Design review of the part shown in the three views and the two pictorial views. Dimensions are in mm from the part's minimum x, y and z. Coordinates: 2 decimals unless noted, no trailing zeros. Loops run counter-clockwise (first coordinate to the right, second up) from the corner with the lowest first, then second, coordinate; pieces in that order, holes last. Notation, with made-up numbers: M -26.75,68.5 L -1.75,68.5 A25 cw -1.75,87.5 Z; hole C 86,-33 d6. An arc over 180 degrees is marked long. Answer as a JSON object with one key per item and string values. Group by question number.
Item 1: Wall thickness on L1, parallel to X at y = 58.5, z = 42.5: over which ranges is the line inside the solid? List them lowest first. Write a range as from..to.
Item 2: Add section A-A (x = 12.5). State the section outline as (y, z) points, then the cut area to 3 significant figures.
Item 3: Add section C-C (z = 40). State the section outline as (x, y) points, then the cut area to 3 significant figures.
Item 4: Add section B-B (y = 29). State the section outline as (x, z) points, then the cut area to 3 significant figures.
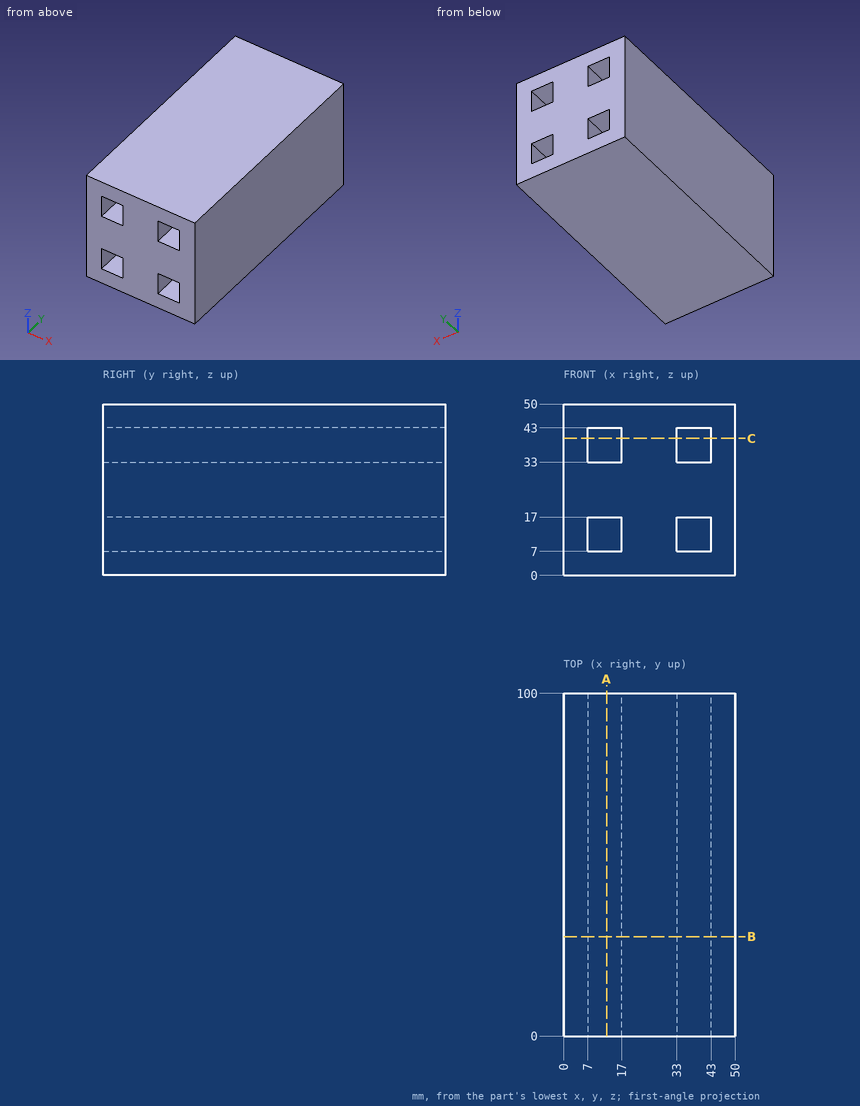
From the geometry:
{
 "1": {"L1": "x = 0..7, 17..33, 43..50"},
 "2": {"outline": "M 0,0 L 100,0 L 100,7 L 0,7 Z; M 0,17 L 100,17 L 100,33 L 0,33 Z; M 0,43 L 100,43 L 100,50 L 0,50 Z", "area": "3,000 mm²"},
 "3": {"outline": "M 0,0 L 7,0 L 7,100 L 0,100 Z; M 17,0 L 33,0 L 33,100 L 17,100 Z; M 43,0 L 50,0 L 50,100 L 43,100 Z", "area": "3,000 mm²"},
 "4": {"outline": "M 0,0 L 50,0 L 50,50 L 0,50 Z; hole M 7,7 L 17,7 L 17,17 L 7,17 Z; hole M 7,33 L 17,33 L 17,43 L 7,43 Z; hole M 33,7 L 43,7 L 43,17 L 33,17 Z; hole M 33,33 L 43,33 L 43,43 L 33,43 Z", "area": "2,100 mm²"}
}
